Could you check a few things on this model? Use its own coordinates, in mm. A direction names the side the tool comes from. Give positions to 0.01 mm unless a question says otherwise; leave off trailing zeros. Write each loop counter-clockwise with the first axis right and the second up, starting at its lowest first coordinate (ties: lowest second). Pieces come first, ordered by that corner, then holes. Notation, with made-up numbers: M 63,-0.5 L 92,-0.5 A23 cw 92,33.5 Z; hole C 83,30.25 d2. An arc over 180 degrees is marked long. One line per item, written item: value.
```python
from build123d import *

# Parameters (mm, degrees)
F1_DEPTH  = 1
F2_W      = 60
F2_H      = 16
F2_W_2    = 58
F2_H_2    = 14
F3_DEPTH  = 10
F4_R      = 1.5
F5_DEPTH  = 20
F8_DEPTH  = 0.5
F11_W     = 11
F11_H     = 3
F12_DEPTH = 2.0010001


with BuildPart() as f1:
    # F0 (on Top) → F1 (new body, symmetric)
    with BuildSketch(Plane.XY):
        with BuildLine():
            Line((-48.5, 8.5), (-48.5, 0))
            Line((-48.5, 0), (-48.5, -8.5))
            ThreePointArc((-48.5, -8.5), (-47.0355339059, -12.0355339059), (-43.5, -13.5))
            Line((-43.5, -13.5), (-1.5, -13.5))
            Line((-1.5, -13.5), (-1.5, -11))
            ThreePointArc((-1.5, -11), (0, -9.5), (1.5, -11))
            Line((1.5, -11), (1.5, -13.5))
            ThreePointArc((1.5, -13.5), (29.3474128971, -15.612168306), (54.6807093507, -3.8578605504))
            ThreePointArc((54.6807093507, -3.8578605504), (56.5, 0), (54.6807093507, 3.8578605504))
            ThreePointArc((54.6807093507, 3.8578605504), (29.3474128971, 15.612168306), (1.5, 13.5))
            Line((1.5, 13.5), (1.5, 11))
            ThreePointArc((1.5, 11), (0, 9.5), (-1.5, 11))
            Line((-1.5, 11), (-1.5, 13.5))
            Line((-1.5, 13.5), (-43.5, 13.5))
            ThreePointArc((-43.5, 13.5), (-47.0355339059, 12.0355339059), (-48.5, 8.5))
        make_face()
    extrude(amount=F1_DEPTH, both=True)

    # F2 (on face) → F3 (join)
    with BuildSketch(Plane.XY.offset(1)):
        with Locations((-3.5, 0)):
            Rectangle(F2_W, F2_H)
        with Locations((-3.5, 0)):
            Rectangle(F2_W_2, F2_H_2, mode=Mode.SUBTRACT)
    extrude(amount=F3_DEPTH)

    # F4 (on face) → F5 (join)
    with BuildSketch(Plane.XZ.offset(8)):
        with Locations((-8, 0.5)):
            Circle(F4_R)
        with Locations((8, 0.5)):
            Circle(F4_R)
    extrude(amount=F5_DEPTH)



with BuildPart() as f8:
    # F7 (on offset) → F8 (new body, symmetric)
    with BuildSketch(Plane.YZ.offset(-8)):
        Polygon((-8, 7), (-22, 3), (-22, 0), (-8, 0), align=None)
    extrude(amount=F8_DEPTH, both=True)


with BuildPart() as f1_1:
    add(f1.part)

    add(f8.part)  # F9 merges F8
    # F9: F8 across plane
    add(f8.part.mirror(Plane.YZ))

    # F10: F1 across plane


with BuildPart() as f1_2:
    add(f1_1.part)
    add(f1_1.part.mirror(Plane.XZ))

    # F11 (on face) → F12 (cut, through all)
    with BuildSketch(Plane.XY.offset(1)):
        with Locations((25, 9.5)):
            Rectangle(F11_W, F11_H)
        with BuildLine():
            ThreePointArc((-11, 5), (-10.7071067812, 4.2928932188), (-10, 4))
            Line((-10, 4), (-2, 4))
            ThreePointArc((-2, 4), (-1.2928932188, 4.2928932188), (-1, 5))
            Line((-1, 5), (-1, 7))
            Line((-1, 7), (-11, 7))
            Line((-11, 7), (-11, 5))
        make_face()
        with BuildLine():
            ThreePointArc((-10, -4), (-10.7071067812, -4.2928932188), (-11, -5))
            Line((-11, -5), (-11, -7))
            Line((-11, -7), (-1, -7))
            Line((-1, -7), (-1, -5))
            ThreePointArc((-1, -5), (-1.2928932188, -4.2928932188), (-2, -4))
            Line((-2, -4), (-10, -4))
        make_face()
        with Locations((25, -9.5)):
            Rectangle(F11_W, F11_H)
    extrude(amount=-F12_DEPTH, mode=Mode.SUBTRACT)


solid = f1_2.part
```
1) If we section it at A-A, the plane x = -4.5: Write out the boundary of the cut face in (y, z), then the cut area to 3 significant figures.
Outcome:
outline: M -13.5,-1 L -7,-1 L -7,11 L -8,11 L -8,1 L -13.5,1 Z; M -4,-1 L 4,-1 L 4,1 L -4,1 Z; M 7,-1 L 13.5,-1 L 13.5,1 L 8,1 L 8,11 L 7,11 Z
area: 62.0 mm^2
2) On a 3-axis mill with a long thin cutter (end or side, diameter ignored), from which of +Z, -Z, +X, -X, +Y, -Y can I reach the whole of each face in a straight line? I mean faces 1 (the face through (-1, -6, 0)), 2 (the face through (-1.5, -12, 0)), 3 (the face through (6.89, -20.08, 1.51)). Say none if no direction works.
Outcome:
face 1: +Z, -Z
face 2: +Z, -Z, -Y
face 3: -Y
3) Please list where these lines run through material, in increasing order: L1, parallel to X at y = 14, z = 4.75; L2, parallel to Y at x = -20.5, z = 4; L3, parallel to Z at x = -41, y = -8.5. Write a range as from..to.
Outcome:
L1: x = -8.5..-7.5, 7.5..8.5
L2: y = -8..-7, 7..8
L3: z = -1..1
4) I'm going to push flat-ended pins straight in: pin 1 (1.5 mm diameter, centred on y = 14, z = 4.5, fed in from -X); pin 2 (1.6 mm diameter, centred on y = 5.5, z = 0.5, fed in from +X); pin 3 (1 mm diameter, centred on y = -11.5, z = 0, fed in from +X); pin 4 (8 mm diameter, centred on x = 17.5, y = -17, fed in from -Z). Where does each tip first touch, or does it pass through?
Outcome:
pin 1: stops at x = -8.5
pin 2: stops at x = 53.63
pin 3: stops at x = 43.53
pin 4: stops at z = -1
5) We'd pull the mould along Y, two halves only. Please class faces 4 (the face through (30.5, 9, 0)), 5 (the face through (-7.5, -14, 4)), 6 (the face through (-8, 28, 1)): pulls with the +Y half, pulls with the -Y half, needs draft (parallel to the pull), parting line crosses it, or undercut.
Outcome:
face 4: undercut
face 5: needs draft
face 6: pulls with the +Y half
6) If we section it at D-D, the plane x = -35: Write out the boundary of the cut face in (y, z).
Outcome:
outline: M -13.5,-1 L 13.5,-1 L 13.5,1 L -13.5,1 Z
7) If we section it at C-C, the plane y = 25.5: Write out the boundary of the cut face in (x, z), then the cut area to 3 significant figures.
Outcome:
outline: C -8,0.5 d3; C 8,0.5 d3
area: 14.1 mm^2
8) If we section it at B-B, the plane z = 8: Write out the boundary of the cut face in (x, y).
Outcome:
outline: M -33.5,-8 L 26.5,-8 L 26.5,8 L -33.5,8 Z; hole M -32.5,-7 L 25.5,-7 L 25.5,7 L -32.5,7 Z
